Could you check a few things on this model? Use its own coordinates, in mm. Give positions to 0.01 mm unless a question says otherwise; leave off trailing zeros. Order: outer loops, then holes, each group sorted by start corner. A loop starts at its lowest first (then second) coordinate and runs counter-clockwise, first axis right, second up. Notation, with made-up numbers: (4, 68.25) - (33, 68.25) arc R20 cw to (33, 94.25) - close; hole circle Ø8 at (-3, 54.25). An arc over 180 degrees is marked (long way). One line per question, with ' | ' between items. Start each with the question number.
1. For P1, Ø4, axis at x = 8.4, z = -16.575, coming from the -Y side, with a flat end and sliding along its axis, tell me the tip position at first contact or that it passes through.
2. Imagine slicing it at C-C (z = 22). Please give me the cut outline in (x, y).
3. Imagine slicing it at A-A (x = -12.7). Please give me the cut outline in (y, z) (3 decimals).
4. Imagine slicing it at D-D (x = 8.4). Please give me the cut outline in (y, z) (3 decimals).
5. I need wall thicknesses on probe 1 along Z at (x, y) = (-12.7, 2.1) (3 decimals); probe 2 along Z at (x, y) = (8.4, 3.1) (3 decimals). Which ranges of each line are inside material? Lowest first, please. Write a range as from..to.
6. If we mould it in two halves opening along X, with no side actions, what happens to faces 1 (the flat face through (0, 5.08, 0)), 2 (the flat face through (25.4, 3, 0)), 3 (the cylindrical face through (6.302, 2.504, 16.667))? For each: released by +X, released by -X, zero draft, split by the parting line, or undercut.
7. Imagine slicing it at B-B (y = 3.2). Please give me the cut outline in (x, z) (1 decimal).
```python
from build123d import *

# Parameters (mm, degrees)
SKETCH1_W           = 50.8
SKETCH1_H           = 57.15
BOSS_EXTRUDE1_DEPTH = 5.08
SKETCH2_R           = 4.7625
CUT_EXTRUDE1_DEPTH  = 5.08
SKETCH3_R           = 2.1
CUT_EXTRUDE3_DEPTH  = 6.08


with BuildPart() as part:
    # Sketch1 → Boss-Extrude1 (new body)
    with BuildSketch(Plane(origin=(0, 0, 0), x_dir=(1, 0, 0), z_dir=(0, 1, 0))):
        Rectangle(SKETCH1_W, SKETCH1_H)
    extrude(amount=BOSS_EXTRUDE1_DEPTH)

    # Sketch2 → Cut-Extrude1 (cut)
    with BuildSketch(Plane(origin=(0, 5.08, 0), x_dir=(1, 0, 0), z_dir=(0, 1, 0))):
        with Locations((-12.7, 18.837656)):
            Circle(SKETCH2_R)
        with Locations((-12.7, -18.837656)):
            Circle(SKETCH2_R)
    extrude(amount=-CUT_EXTRUDE1_DEPTH, mode=Mode.SUBTRACT)

    # Sketch3 → Cut-Extrude3 (cut, through all)
    with BuildSketch(Plane.XZ):
        with Locations((8.4, -16.575)):
            Circle(SKETCH3_R)
        with Locations((8.4, 16.575)):
            Circle(SKETCH3_R)
    extrude(amount=-CUT_EXTRUDE3_DEPTH, mode=Mode.SUBTRACT)


solid = part.part
```
Results found:
1) P1: passes through
2) outline: (-25.4, 0) - (-16.26, 0) - (-16.26, 5.08) - (-25.4, 5.08) - close; (-9.14, 0) - (25.4, 0) - (25.4, 5.08) - (-9.14, 5.08) - close
3) outline: (0, -28.575) - (5.08, -28.575) - (5.08, -23.6) - (0, -23.6) - close; (0, -14.075) - (5.08, -14.075) - (5.08, 14.075) - (0, 14.075) - close; (0, 23.6) - (5.08, 23.6) - (5.08, 28.575) - (0, 28.575) - close
4) outline: (0, -28.575) - (5.08, -28.575) - (5.08, -18.675) - (0, -18.675) - close; (0, -14.475) - (5.08, -14.475) - (5.08, 14.475) - (0, 14.475) - close; (0, 18.675) - (5.08, 18.675) - (5.08, 28.575) - (0, 28.575) - close
5) probe 1: z = -28.575..-23.6, -14.075..14.075, 23.6..28.575 | probe 2: z = -28.575..-18.675, -14.475..14.475, 18.675..28.575
6) face 1: zero draft | face 2: released by +X | face 3: undercut
7) outline: (-25.4, -28.6) - (25.4, -28.6) - (25.4, 28.6) - (-25.4, 28.6) - close; hole circle Ø9.5 at (-12.7, -18.8); hole circle Ø9.5 at (-12.7, 18.8); hole circle Ø4.2 at (8.4, -16.6); hole circle Ø4.2 at (8.4, 16.6)
